Verification items for the finished model (mm, model axes). A direction names the side the tool comes from. Round coordinates to 2 decimals unless told otherwise and drop trailing zeros. Write each loop counter-clockwise with the first axis right and the second up, starting at its lowest first coordinate (ties: lowest second). Pieces come first, ordered by that corner, then holes. Notation, with made-up numbers: (54, 20.5) -> (66, 20.5) arc R21 cw to (66, 41.5) -> close; hole circle Ø7 at (-27.75, -25). An arc over 180 degrees is marked (long way). Answer as a JSON object with one key per item and string values. Group by question number.
(1) Scan lines: L1, parallel to X at y = -4, z = -25.4; L2, parallel to Z at x = -2.5, y = 0.25 (3 decimals); L3, parallel to X at y = 4.5, z = 2.5 (3 decimals). Record each from-to range of solid material in increasing order. Write a range as from..to.
(2) Sectioned sample at A-A on z = -25.4. Record the cut outline in (x, y).
(3) Sectioned sample at D-D on x = 5.75. Record the cut outline in (y, z).
(4) Gauge pin test, flat ends, axial feed: pin 1 Ø0.6 at (x, y) = (0, 0) entering from +Z; pin 2 Ø6 at (x, y) = (6.5, 3.5) entering from +Z; pin 3 Ø1.2 at (x, z) = (1, 6.5) entering from +Y (3 decimals). Record the tip position at first contact, or that the pin passes through.
(5) Sectioned sample at B-B on x = 0. Count the separate pieces of the cut face and the enclosed holes in it, and give its area (3 significant figures).
(6) Draft check along X on faces 4 (the face through (0.635, 2, -37)), 5 (the face through (2, 0, 9.525)), 6 (the face through (-3.175, 0, -4)), 7 (the face through (1.626, 0, 8)). Enter one of: released by +X, released by -X, zero draft, split by the parting line, or undercut.
(7) Sectioned sample at C-C on y = 5. Record the cut outline in (x, z) (3 decimals), and give its area (3 significant figures).
(8) Set-up check for faces 1 (the face through (-1.626, 0, 8)), 2 (the face through (0, -3.175, 6)), 3 (the face through (-0.635, 2, -37)): record each of +Z, -Z, +X, -X, +Y, -Y from which the full face is reachable in a straight line by a thin tool's end or side.
```python
from build123d import *

# Parameters (mm, degrees)
SKETCH1_R               = 3.302
BOSS_EXTRUDE1_DEPTH     = 3.175
SKETCH2_R               = 12.7
BOSS_EXTRUDE2_DEPTH     = 12.7
CUT_EXTRUDE1_REACH      = 44.121
SKETCH3_R               = 3.556
SKETCH4_R               = 9.921875
CUT_EXTRUDE2_DEPTH      = 6.35
CUT_EXTRUDE3_REACH      = 51.697
CUT_EXTRUDE3_END_RADIUS = 9.921875
SKETCH5_W               = 1.27
SKETCH5_H               = 3.2004
SKETCH6_W               = 3.2512
SKETCH6_H               = 1.27
CUT_EXTRUDE4_DEPTH      = 3.175
FILLET2_R               = 2.54


with BuildPart() as part:
    # Sketch1 → Boss-Extrude1 (new, symmetric)
    with BuildSketch(Plane(origin=(0, 0, 0), x_dir=(0, 0, -1), z_dir=(1, 0, 0))):
        with BuildLine():
            Line((0, -6.35), (38.1, -6.35))
            Line((38.1, -6.35), (38.1, 6.35))
            Line((38.1, 6.35), (0, 6.35))
            ThreePointArc((0, 6.35), (-3.175, 5.499261314), (-5.499261314, 3.175))
            Line((-5.499261314, 3.175), (-9.525, 3.175))
            Line((-9.525, 3.175), (-9.525, -3.175))
            Line((-9.525, -3.175), (-5.499261314, -3.175))
            ThreePointArc((-5.499261314, -3.175), (-3.175, -5.499261314), (0, -6.35))
        make_face()
        Circle(SKETCH1_R, mode=Mode.SUBTRACT)
    extrude(amount=BOSS_EXTRUDE1_DEPTH, both=True)

    # Sketch2 → Boss-Extrude2 (add)
    with BuildSketch(Plane(origin=(0, 6.35, 0), x_dir=(1, 0, 0), z_dir=(0, 1, 0))):
        with Locations((0, 25.4)):
            Circle(SKETCH2_R)
    extrude(amount=-BOSS_EXTRUDE2_DEPTH)

    # Sketch3 → Cut-Extrude1 (cut, up to next)
    with BuildSketch(Plane.XZ.offset(6.35), mode=Mode.PRIVATE) as cut_extrude1_sk1:
        with Locations(Location((0, -25.4, 0), (0, 0, 270))):
            Circle(SKETCH3_R)
    cut_extrude1_tool1 = extrude(cut_extrude1_sk1.sketch, amount=-CUT_EXTRUDE1_REACH, mode=Mode.PRIVATE) & part.part
    add(cut_extrude1_tool1.solids().sort_by_distance((0, -6.35, -25.4))[0], mode=Mode.SUBTRACT)

    # Sketch4 → Cut-Extrude2 (cut)
    with BuildSketch(Plane.XZ.offset(6.35)):
        with Locations(Location((0, -25.4, 0), (0, 0, 270))):
            Circle(SKETCH4_R)
    extrude(amount=-CUT_EXTRUDE2_DEPTH, mode=Mode.SUBTRACT)

    # Cut-Extrude3: up to this cylinder (the profile starts outside it)
    cut_extrude3_end = Plane(origin=(0, 1.5748, -25.4), z_dir=(0, -1, 0)) * Cylinder(CUT_EXTRUDE3_END_RADIUS, 124.23775, mode=Mode.PRIVATE)
    # Sketch5 → Cut-Extrude3 (cut, up to the surface)
    with BuildSketch(Plane(origin=(0, 0, -38.1), x_dir=(-1, 0, 0), z_dir=(0, 0, -1)), mode=Mode.PRIVATE) as cut_extrude3_sk1:
        with Locations((0, 1.5748)):
            Rectangle(SKETCH5_W, SKETCH5_H)
    cut_extrude3_tool1 = extrude(cut_extrude3_sk1.sketch, amount=-CUT_EXTRUDE3_REACH, mode=Mode.PRIVATE) - cut_extrude3_end
    add(cut_extrude3_tool1.solids().sort_by_distance((0, 1.5748, -38.1))[0], mode=Mode.SUBTRACT)

    # Sketch6 → Cut-Extrude4 (cut)
    with BuildSketch(Plane.XY.offset(9.525)):
        Rectangle(SKETCH6_W, SKETCH6_H)
    extrude(amount=-CUT_EXTRUDE4_DEPTH, mode=Mode.SUBTRACT)

    # Fillet2
    fillet2_edges = [part.edges().sort_by_distance(p)[0] for p in [
        (0, -3.175, 9.525),
        (0, 3.175, 9.525),
    ]]
    fillet(fillet2_edges, radius=FILLET2_R - 0.0001)  # a hair under: the kernel refuses the full size


solid = part.part
```
Computed values:
{
 "1": {"L1": "-12.7..-9.92, 9.92..12.7", "L2": "-38.1..-27.929, -22.871..-3.293, 3.293..9.525", "L3": "-3.175..3.175"},
 "2": {"outline": "(-12.7, -6.35) -> (-9.92, -6.35) -> (-9.92, 0) -> (-3.56, 0) -> (-3.56, 6.35) -> (-12.7, 6.35) -> close; (3.56, 0) -> (9.92, 0) -> (9.92, -6.35) -> (12.7, -6.35) -> (12.7, 6.35) -> (3.56, 6.35) -> close"},
 "3": {"outline": "(-6.35, -36.72) -> (6.35, -36.72) -> (6.35, -14.08) -> (-6.35, -14.08) -> (-6.35, -17.31) -> (0, -17.31) -> (0, -33.49) -> (-6.35, -33.49) -> close"},
 "4": {"pin 1": "z = 6.35", "pin 2": "z = -13.19", "pin 3": "y = 3.175"},
 "5": {"separate pieces": "3", "enclosed holes": "1", "area": "348 mm2"},
 "6": {"face 4": "undercut", "face 5": "zero draft", "face 6": "released by -X", "face 7": "undercut"},
 "7": {"outline": "(-3.175, -38.1) -> (3.175, -38.1) -> (3.175, -37.697) arc R12.7 ccw to (3.175, -13.103) -> (3.175, 3.914) -> (-3.175, 3.914) -> (-3.175, -13.103) arc R12.7 ccw to (-3.175, -37.697) -> close; hole circle Ø7.112 at (0, -25.4)", "area": "574 mm2"},
 "8": {"face 1": "+Z", "face 2": "+Z, +X, -X, -Y", "face 3": "-Z"}
}
